Could you check a few things on this model? Use its own coordinates, in mm. A direction names the side the tool comes from. Give positions to 0.01 mm unless a question says otherwise; leave off trailing zeros. Order: outer loops, then holes, each group sorted by start corner. A loop starts at its lowest first (then second) coordinate and runs counter-clockwise, first axis right, second up. Notation, with made-up numbers: M 70.5,-9 L 75.5,-9 A11 cw 75.5,9 Z; hole C -19.5,-22.75 d6. An arc over 180 degrees is marked long. Answer in a Markdown table with one row per item. Add a question column.
```python
from build123d import *

# Parameters (mm, degrees)
F0_W     = 106
F0_H     = 57.8
F0_R     = 3.75
F0_R_2   = 14.5
F1_DEPTH = 6
F3_DEPTH = 6
F4_D     = 3.3
F5_R     = 5


with BuildPart() as f1:
    # F0 (on Front) → F1 (new body)
    with BuildSketch(Plane.XZ):
        with Locations((53, 28.9)):
            Rectangle(F0_W, F0_H)
        with Locations((53.2, 9.2)):
            Circle(F0_R, mode=Mode.SUBTRACT)
        with Locations((83.2, 9.2)):
            Circle(F0_R, mode=Mode.SUBTRACT)
        with Locations((68.2, 24.2)):
            Circle(F0_R_2, mode=Mode.SUBTRACT)
        with Locations((53.2, 39.2)):
            Circle(F0_R, mode=Mode.SUBTRACT)
        with Locations((83.2, 39.2)):
            Circle(F0_R, mode=Mode.SUBTRACT)
    extrude(amount=F1_DEPTH)

    # F2 (on face) → F3 (cut, through all)
    with BuildSketch(Plane.XZ.offset(6)):
        with BuildLine():
            Line((7.8, 54.5), (5.8, 54.5))
            ThreePointArc((5.8, 54.5), (3.3, 52), (5.8, 49.5))
            Line((5.8, 49.5), (7.8, 49.5))
            ThreePointArc((7.8, 49.5), (10.3, 52), (7.8, 54.5))
        make_face()
        with BuildLine():
            Line((7.8, 8.3), (5.8, 8.3))
            ThreePointArc((5.8, 8.3), (3.3, 5.8), (5.8, 3.3))
            Line((5.8, 3.3), (7.8, 3.3))
            ThreePointArc((7.8, 3.3), (10.3, 5.8), (7.8, 8.3))
        make_face()
        with BuildLine():
            Line((100.2, 8.3), (98.2, 8.3))
            ThreePointArc((98.2, 8.3), (95.7, 5.8), (98.2, 3.3))
            Line((98.2, 3.3), (100.2, 3.3))
            ThreePointArc((100.2, 3.3), (102.7, 5.8), (100.2, 8.3))
        make_face()
        with BuildLine():
            Line((100.2, 54.5), (98.2, 54.5))
            ThreePointArc((98.2, 54.5), (95.7, 52), (98.2, 49.5))
            Line((98.2, 49.5), (100.2, 49.5))
            ThreePointArc((100.2, 49.5), (102.7, 52), (100.2, 54.5))
        make_face()
    extrude(amount=-F3_DEPTH, mode=Mode.SUBTRACT)

    # F4 (through all)
    with Locations(Plane.XZ.offset(6)):
        with Locations((51.7, 29.3), (84.7, 29.3)):
            Hole(F4_D / 2)

    # F5
    f5_edges = [f1.edges().sort_by_distance(p)[0] for p in [
        (106, -3, 57.8),
        (106, -3, 0),
        (0, -3, 0),
        (0, -3, 57.8),
    ]]
    fillet(f5_edges, radius=F5_R)


solid = f1.part
```
1. Thinking about a two-plate mould opening in Z: for faces 1 (the cylindrical face through (95.7, -3, 52.1)), 2 (the flat face through (106, -3, 29)), 3 (the cylindrical face through (104.5, -3.04, 56.37)), which applies, pulls with the +Z half, pulls with the -Z half, needs draft (parallel to the pull), parting line crosses it, or undercut?
2. Suppose I cut it at C-C on z = 32. List the corners of the cut face in (x, y) for me, plus the area to 3 significant figures.
3. If I drill on line 1 along X through (y, z) = (-3.55, 9); line 2 along Z through (x, y) = (81.5, -3.6); line 3 along Z through (x, y) = (83.2, -3.35), over which ranges is the centre line in solid material (lowest first)? Write a range as [from, to].
4. For faces 4 (the flat face through (7, -3, 49.5)), 5 (the cylindrical face through (104, -3, 1)), which set-ups out of +Z, -Z, +X, -X, +Y, -Y let a thin tool reach every point of the face, with its end or its side?
5. Suppose I cut it at B-B on y = -1.6. Count the separate pieces of the cut face and the enclosed holes in it, plus the area to 3 significant figures.
6. Suppose I cut it at D-D on x = 55. List the corners of the cut face in (y, z) for me, plus the area to 3 significant figures.
7. Suppose I cut it at A-A on x = 68.2. List the corners of the cut face in (y, z) for me, plus the area to 3 significant figures.
Findings below:
| question | item | result |
|---|---|---|
| 1 | face 1 | undercut |
| 1 | face 2 | needs draft |
| 1 | face 3 | pulls with the +Z half |
| 2 | outline | M 0,-6 L 55.98,-6 L 55.98,0 L 0,0 Z; M 80.42,-6 L 106,-6 L 106,0 L 80.42,0 Z |
| 2 | area | 489 mm2 |
| 3 | line 1 | [0, 49.46], [56.94, 79.46], [86.94, 106] |
| 3 | line 2 | [0, 5.86], [12.54, 18.42], [29.98, 35.86], [42.54, 57.8] |
| 3 | line 3 | [0, 5.45], [12.95, 28.61], [29.99, 35.45], [42.95, 57.8] |
| 4 | face 4 | +Y, -Y |
| 4 | face 5 | -Z, +X, +Y, -Y |
| 5 | separate pieces | 1 |
| 5 | enclosed holes | 11 |
| 5 | area | 5,130 mm2 |
| 6 | outline | M -6,0 L 0,0 L 0,5.91 L -6,5.91 Z; M -6,12.49 L 0,12.49 L 0,18.2 L -6,18.2 Z; M -6,30.2 L 0,30.2 L 0,35.91 L -6,35.91 Z; M -6,42.49 L 0,42.49 L 0,57.8 L -6,57.8 Z |
| 6 | area | 196 mm2 |
| 7 | outline | M -6,0 L 0,0 L 0,9.7 L -6,9.7 Z; M -6,38.7 L 0,38.7 L 0,57.8 L -6,57.8 Z |
| 7 | area | 173 mm2 |
